The listing builds one solid part. Answer for the finished solid, in the listing's coordinates (mm). A direction names the side the tool comes from. Round coordinates to 2 decimals unless told otherwise and drop trailing zeros. Write each loop counter-clockwise with the first axis right and the second up, starting at its lowest first coordinate (ties: lowest second). Pieces come first, ordered by that corner, then holes.
(1) A cutting plane is placed at A-A, the plane z = -63.5. Give the vertices of the cut face in (x, y), and give its area (3 significant figures).
(2) Each of these flat-tipped pins is pushed along its axis until it touches: pin 1 Ø1.5 at (x, y) = (39, -67.5) entering from +Z; pin 2 Ø12 at (x, z) = (54.5, -33) entering from -Y. Where does it stop, or does it pass through?
(3) A cutting plane is placed at C-C, the plane z = 0. Give the vertices of the cut face in (x, y), and give its area (3 significant figures).
(4) A cutting plane is placed at D-D, the plane x = 0. Give the vertices of the cut face in (y, z), and give its area (3 significant figures).
(5) A cutting plane is placed at B-B, the plane x = -54.5. Give the vertices of the cut face in (y, z).
(6) The mould has two halves that part along Z. Classify faces 5 (the face through (-1, -50, 76.2)), 6 (the face through (-7.709, -418.211, -98.214)), 7 (the face through (-1, -355.6, 2)), 8 (the face through (-6.883, -126.644, -30.995)): +Z half, -Z half, draft (parallel to the pull), parting line (faces both ways), or undercut.
(7) For faces 1 (the face through (-76.2, -253, -2)), 2 (the face through (-7.709, -418.211, 28.786)), 3 (the face through (-1, -50, -76.2)), 4 (the face through (-18, -152.4, 30)), determine the directions among +Z, -Z, +X, -X, +Y, -Y from which every point of the face is accessible in a straight line to the end or side of a thin tool.
(8) Find the intervals of material crossed by probe 1 along Y at (x, z) = (37.5, -37.5); probe 2 along Y at (x, z) = (43.5, 100); probe 3 along X at (y, z) = (-371, -62), in increasing order.
from build123d import *

# Parameters (mm, degrees)
F0_W     = 152.4
F0_H     = 152.4
F1_DEPTH = 101.6
F2_R     = 31.75
F3_DEPTH = 50.8
F4_W     = 152.4
F4_H     = 254
F5_DEPTH = 203.2
F6_R     = 35.56
F7_DEPTH = 127


with BuildPart() as f1:
    # F0 (on Front) → F1 (new body)
    with BuildSketch(Plane.XZ):
        Rectangle(F0_W, F0_H)
    extrude(amount=F1_DEPTH)

    # F2 (on face) → F3 (join)
    with BuildSketch(Plane.XZ.offset(101.6)):
        Circle(F2_R)
    extrude(amount=F3_DEPTH)

    # F4 (on face) → F5 (join)
    with BuildSketch(Plane.XZ.offset(152.4)):
        Rectangle(F4_W, F4_H)
    extrude(amount=F5_DEPTH)

    # F6 (on face) → F7 (join)
    with BuildSketch(Plane.XZ.offset(355.6)):
        with Locations((0, -63.5)):
            Circle(F6_R)
        with Locations((0, 63.5)):
            Circle(F6_R)
    extrude(amount=F7_DEPTH)


solid = f1.part
Solutions:
1. outline: (-76.2, -355.6) - (-35.56, -355.6) - (-35.56, -482.6) - (35.56, -482.6) - (35.56, -355.6) - (76.2, -355.6) - (76.2, -152.4) - (-76.2, -152.4) - close; (-76.2, -101.6) - (76.2, -101.6) - (76.2, 0) - (-76.2, 0) - close
1. area: 55,500 mm2
2. pin 1: stops at z = 76.2
2. pin 2: stops at y = -355.6
3. outline: (-76.2, -355.6) - (76.2, -355.6) - (76.2, -152.4) - (31.75, -152.4) - (31.75, -101.6) - (76.2, -101.6) - (76.2, 0) - (-76.2, 0) - (-76.2, -101.6) - (-31.75, -101.6) - (-31.75, -152.4) - (-76.2, -152.4) - close
3. area: 49,700 mm2
4. outline: (-482.6, -99.06) - (-355.6, -99.06) - (-355.6, -127) - (-152.4, -127) - (-152.4, -31.75) - (-101.6, -31.75) - (-101.6, -76.2) - (0, -76.2) - (0, 76.2) - (-101.6, 76.2) - (-101.6, 31.75) - (-152.4, 31.75) - (-152.4, 127) - (-355.6, 127) - (-355.6, 99.06) - (-482.6, 99.06) - (-482.6, 27.94) - (-355.6, 27.94) - (-355.6, -27.94) - (-482.6, -27.94) - close
4. area: 88,400 mm2
5. outline: (-355.6, -127) - (-152.4, -127) - (-152.4, 127) - (-355.6, 127) - close; (-101.6, -76.2) - (0, -76.2) - (0, 76.2) - (-101.6, 76.2) - close
6. face 5: +Z half
6. face 6: undercut
6. face 7: undercut
6. face 8: parting line
7. face 1: +Z, -Z, -X, +Y, -Y
7. face 2: -Y
7. face 3: -Z, +X, -X, +Y
7. face 4: none
8. probe 1: y = -355.6 to -152.4, -101.6 to 0
8. probe 2: y = -355.6 to -152.4
8. probe 3: x = -35.53 to 35.53
